Geometry check sheet. Reference: the model listing, model coordinates, mm. Face numbers are marked on the shaded views. Round coordinates to 2 decimals unless told otherwise and drop trailing zeros. Order: outer loops, then holes, each group sorted by start corner. A loop starts at its lowest first (then second) coordinate and runs counter-clockwise, first axis right, second up. Notation, with made-up numbers: (-19, -8.75) -> (15, -8.75) arc R25 ccw to (15, 23.25) -> close; hole circle Ø8 at (0, 85.5). An arc over 180 degrees is marked (long way). Use a Markdown table: item, result. Add a question column.
Item 1: Gauge pin test, flat ends, axial feed: pin 1 Ø8 at (x, z) = (-9.5, 43) entering from -Y; pin 2 Ø6 at (y, z) = (6.5, 41.5) entering from -X; pin 3 Ø1.5 at (x, z) = (14, 20) entering from +Y; pin 4 Ø2 at (x, y) = (11, 20) entering from +Z. Record the tip position at first contact, or that the pin passes through.
Item 2: Sectioned sample at A-A, the plane z = 5. Record the cut outline in (x, y).
Item 3: Mould release check, pull along Y, two halves, no side actions. Record for the marked faces 1 and 2: pulls with the +Y half, pulls with the -Y half, needs draft (parallel to the pull), parting line crosses it, or undercut.
Item 4: Material ranges on probe 1 along Z at (x, y) = (-18, -8.5); probe 2 along X at (y, z) = (0, 9); probe 3 along X at (y, z) = (0, 6.75), recorded low to high. Write a range as [from, to].
Item 5: Sectioned sample at B-B, the plane z = 58.5. Record the cut outline in (x, y).
from build123d import *

# Parameters (mm, degrees)
F2_DEPTH = 12.7
F3_R     = 5.08
F5_R     = 5.08
F6_R     = 5.08


# Not quite as in the source:
# - a fillet or chamfer that OpenCascade refuses, or shapes differently, is made with other operations: its cross-section is extruded or revolved along the edge and cut away or added


with BuildPart() as f1:
    # F0 (on Front) → F1 (revolve)
    with BuildSketch(Plane.XZ):
        with BuildLine():
            Line((6.3432058776, 63.206334895), (0, 63.5))
            Line((0, 63.5), (0, 0))
            Line((0, 0), (2.5480911136, 0))
            Line((2.5480911136, 0), (6.6250329837, 10.4471649975))
            Line((6.6250329837, 10.4471649975), (10.9556252941, 16.1543861032))
            Line((10.9556252941, 16.1543861032), (30.48, 16.1543861032))
            Line((30.48, 16.1543861032), (30.4299078499, 21.4240159839))
            Line((30.4299078499, 21.4240159839), (20.699405237, 21.4240159839))
            ThreePointArc((20.699405237, 21.4240159839), (16.6336106625, 21.5337881018), (12.597086859, 22.0329985023))
            ThreePointArc((12.597086859, 22.0329985023), (4.7528583484, 41.9031506128), (6.3432058776, 63.206334895))
        make_face()
    revolve(axis=Axis((0, 0, 31.75), (0, 0, -1)))

    # F2 (cut): a face of the model
    f2_faces = [f1.faces().sort_by_distance(p)[0] for p in [
        (0, 0, 0),
    ]]
    extrude(f2_faces, amount=-F2_DEPTH, mode=Mode.SUBTRACT)

    # F3
    f3_edges = [f1.edges().sort_by_distance(p)[0] for p in [
        (-10.955625, 0, 16.154386),
        (-30.48, 0, 16.154386),
    ]]
    fillet(f3_edges, radius=F3_R)

    # F4: chamfer of 5.08 on 1 edges, made by hand

    # F4_s1 → F4_t2 (revolve, cut)
    with BuildSketch(Plane.XZ):
        Polygon((30.478195231, 16.3442454843), (25.3499078499, 21.4240159839), (30.4299078499, 21.4240159839), align=None)
    revolve(axis=Axis((0, 0, 21.4240159839), (0, 0, -1)), mode=Mode.SUBTRACT)

    # F5
    f5_edges = [f1.edges().sort_by_distance(p)[0] for p in [
        (-20.699405, 0, 21.424016),
        (-12.597087, 0, 22.032999),
        (16.633611, 0, 21.533788),
    ]]
    fillet(f5_edges, radius=F5_R)

    # F6
    f6_edges = [f1.edges().sort_by_distance(p)[0] for p in [
        (-25.349908, 0, 21.424016),
        (-20.699405, 0, 21.424016),
    ]]
    fillet(f6_edges, radius=F6_R)


solid = f1.part
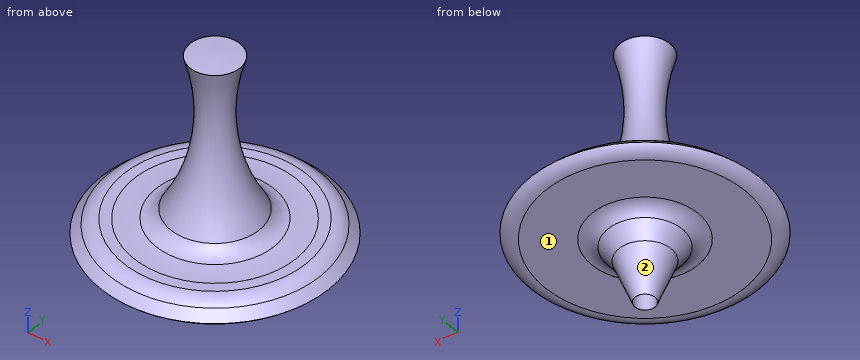
Found:
| question | item | result |
|---|---|---|
| 1 | pin 1 | passes through |
| 1 | pin 2 | stops at x = -3.39 |
| 1 | pin 3 | stops at y = 23.82 |
| 1 | pin 4 | stops at z = 21.42 |
| 2 | outline | circle Ø9 at (0, 0); hole circle Ø5.1 at (0, 0) |
| 3 | face 1 | needs draft |
| 3 | face 2 | parting line crosses it |
| 4 | probe 1 | z = [16.15, 21.41] |
| 4 | probe 2 | x = [-6.06, -2.55], [2.55, 6.06] |
| 4 | probe 3 | x = [-5.18, -2.55], [2.55, 5.18] |
| 5 | outline | circle Ø10.29 at (0, 0) |
